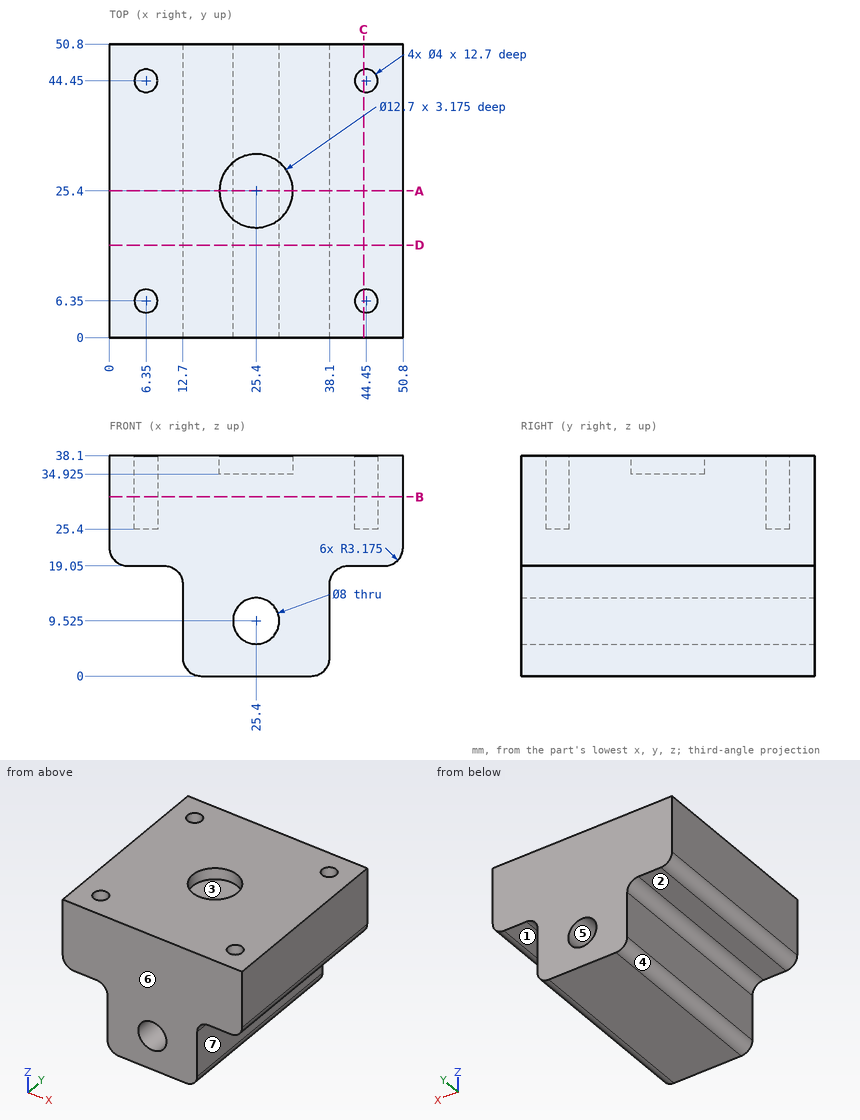
Print and shaded views of the part. All mm, measured from the part's lowest x, y and z. A direction names the side the tool comes from. Coordinates: 2 decimals unless noted, no trailing zeros. Loops run counter-clockwise (first coordinate to the right, second up) from the corner with the lowest first, then second, coordinate; pieces in that order, holes last. Notation, with made-up numbers: (35.5, 1.5) -> (94.5, 1.5) arc R6 ccw to (94.5, 9.5) -> close; hole circle Ø4 at (-4, 30). An arc over 180 degrees is marked (long way). Use a Markdown table: item, result. Add a question column.
Item 1: Probe probe 1 along Y at (x, z) = (6.35, 31.5); probe 2 along X at (y, z) = (45, 34.5); probe 3 along Z at (x, y) = (47, 9). List the from-to ranges inside material, lowest first.
Item 2: Pull direction X, two halves, no side cores. Call the marked faces 4, 5, 6 and 7: +X half, -X half, draft (parallel to the pull), parting line (faces both ways), or undercut.
Item 3: Band-saw the part on D-D on y = 16. Write the cut outline in (x, z) (3 decimals).
Item 4: Band-saw the part on C-C on x = 44. Write the cut outline in (y, z).
Item 5: Band-saw the part on B-B on z = 31. Write the cut outline in (x, y), plus the area to 3 significant figures.
Item 6: Band-saw the part on A-A on y = 25.4. Write the cut outline in (x, z) (3 decimals).
Item 7: Flat gauge pins, fed straight in: P1, Ø2.5, axis at x = 44.45, y = 44.45, coming from the -Z side; P2, Ø1.2, axis at x = 5.5, y = 5.5, coming from the +Z side; P3, Ø4.5, axis at x = 44.5, y = 44, coming from the +Z side; P4, Ø6, axis at y = 18.5, z = 7, coming from the -X side. Where does each tip first touch, or does it go through?
Item 8: Which spindle directions (+Z, -Z, +X, -X, +Y, -Y) get a long thin tool onto all of the face, cutting with end or side? Do the marked faces 1, 2 and 3. Say none if no direction does.
Geometry says:
| question | item | result |
|---|---|---|
| 1 | probe 1 | 0 to 4.35, 8.35 to 42.45, 46.45 to 50.8 |
| 1 | probe 2 | 0 to 4.43, 8.27 to 42.53, 46.37 to 50.8 |
| 1 | probe 3 | 19.05 to 38.1 |
| 2 | face 4 | -X half |
| 2 | face 5 | undercut |
| 2 | face 6 | draft |
| 2 | face 7 | +X half |
| 3 | outline | (0, 22.225) arc R3.175 ccw to (3.175, 19.05) -> (9.525, 19.05) arc R3.175 cw to (12.7, 15.875) -> (12.7, 3.175) arc R3.175 ccw to (15.875, 0) -> (34.925, 0) arc R3.175 ccw to (38.1, 3.175) -> (38.1, 15.875) arc R3.175 cw to (41.275, 19.05) -> (47.625, 19.05) arc R3.175 ccw to (50.8, 22.225) -> (50.8, 38.1) -> (0, 38.1) -> close; hole circle Ø8 at (25.4, 9.525) |
| 4 | outline | (0, 19.05) -> (50.8, 19.05) -> (50.8, 38.1) -> (46.4, 38.1) -> (46.4, 25.4) -> (42.5, 25.4) -> (42.5, 38.1) -> (8.3, 38.1) -> (8.3, 25.4) -> (4.4, 25.4) -> (4.4, 38.1) -> (0, 38.1) -> close |
| 5 | outline | (0, 0) -> (50.8, 0) -> (50.8, 50.8) -> (0, 50.8) -> close; hole circle Ø4 at (6.35, 6.35); hole circle Ø4 at (6.35, 44.45); hole circle Ø4 at (44.45, 6.35); hole circle Ø4 at (44.45, 44.45) |
| 5 | area | 2,530 mm² |
| 6 | outline | (0, 22.225) arc R3.175 ccw to (3.175, 19.05) -> (9.525, 19.05) arc R3.175 cw to (12.7, 15.875) -> (12.7, 3.175) arc R3.175 ccw to (15.875, 0) -> (34.925, 0) arc R3.175 ccw to (38.1, 3.175) -> (38.1, 15.875) arc R3.175 cw to (41.275, 19.05) -> (47.625, 19.05) arc R3.175 ccw to (50.8, 22.225) -> (50.8, 38.1) -> (31.75, 38.1) -> (31.75, 34.925) -> (19.05, 34.925) -> (19.05, 38.1) -> (0, 38.1) -> close; hole circle Ø8 at (25.4, 9.525) |
| 7 | P1 | z = 19.05 |
| 7 | P2 | z = 25.4 |
| 7 | P3 | z = 38.1 |
| 7 | P4 | x = 12.7 |
| 8 | face 1 | -Z, +X, +Y, -Y |
| 8 | face 2 | -Z, -X, +Y, -Y |
| 8 | face 3 | +Z |
